```python
from build123d import *

# Parameters (mm, degrees)
SKETCH1_W           = 38.1
SKETCH1_H           = 152.4
SKETCH1_W_2         = 12.7
SKETCH1_H_2         = 6.35
BOSS_EXTRUDE1_DEPTH = 2.54


with BuildPart() as part:
    # Sketch1 → Boss-Extrude1 (new body)
    with BuildSketch(Plane(origin=(0, 0, 0), x_dir=(1, 0, 0), z_dir=(0, 1, 0))):
        with Locations((19.05, 76.2)):
            Rectangle(SKETCH1_W, SKETCH1_H)
        with Locations((6.35, 155.575)):
            Rectangle(SKETCH1_W_2, SKETCH1_H_2)
        with Locations((31.75, 155.575)):
            Rectangle(SKETCH1_W_2, SKETCH1_H_2)
    extrude(amount=BOSS_EXTRUDE1_DEPTH)


solid = part.part
```
Verification items for the finished model (mm, model axes). A direction names the side the tool comes from. Round coordinates to 2 decimals unless told otherwise and drop trailing zeros. Loops run counter-clockwise (first coordinate to the right, second up) from the corner with the lowest first, then second, coordinate; pieces in that order, holes last. Notation, with made-up numbers: (-40, 49) -> (0, 49) arc R18 ccw to (0, 69) -> close; hole circle Ø7 at (24.5, 41). An arc over 180 degrees is marked (long way). Answer as a JSON object with one key per item and string values.
Q1. Section check A-A (x = 16.5). Record the boundary of the cut face in (y, z), then the cut area to 3 significant figures.
Data:
{"outline": "(0, -152.4) -> (2.54, -152.4) -> (2.54, 0) -> (0, 0) -> close", "area": "387 mm2"}
Q2. Scan line: line 1 (Z direction, x = 13.5, y = 2.4). Record every from-to range of solid material in increasing order. Write a range as from..to.
Data:
{"line 1": "z = -152.4..0"}
Q3. Access from +Z, -Z, +X, -X, +Y, -Y to the whole of each face (thin tool, end or side, straight path). Record for faces 1 (the flat face through (19, 1, -152.4)), 2 (the flat face through (32, 1, -158.75)).
Data:
{"face 1": "-Z, +Y, -Y", "face 2": "-Z, +X, -X, +Y, -Y"}
Q4. Go/stop test with a flat-tipped pin: P1, Ø1.5, axis at y = 2, z = -54, coming from the -X side. Record where the tip stops, or that it passes through.
Data:
{"P1": "stops at x = 0"}
Q5. Draft check along X on faces 3 (the flat face through (19, 2.54, -80)), 4 (the flat face through (38.1, 1, -78)), 5 (the flat face through (25.4, 1, -156)). Enter one of: pulls with the +X half, pulls with the -X half, needs draft (parallel to the pull), parting line crosses it, or undercut.
Data:
{"face 3": "needs draft", "face 4": "pulls with the +X half", "face 5": "undercut"}
